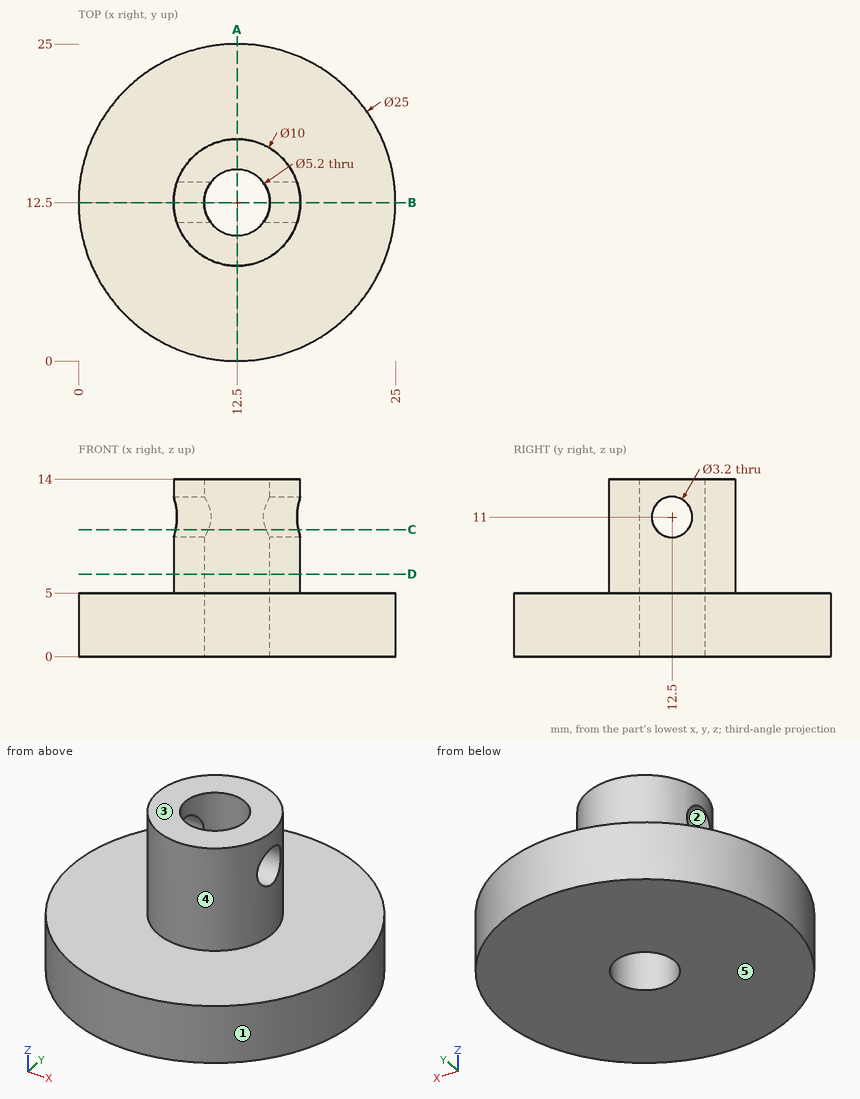
Geometry check sheet. Reference: drawing and pictorial views, mm from the part's lowest x, y, z. A direction names the side the tool comes from. Round coordinates to 2 decimals unless told otherwise and drop trailing zeros. Order: outer loops, then holes, each group sorted by start corner. A loop starts at its lowest first (then second) coordinate and runs counter-clockwise, first axis right, second up. Notation, with made-up numbers: (-21.75, -1) - (-0.75, -1) arc R5 ccw to (-0.75, 8) - close; hole circle Ø5 at (-24.5, 58). An arc over 180 degrees is marked (long way). One line per question, with ' | ' between items. Start each with the question number.
(1) Sectioned sample at D-D on z = 6.5. Record the cut outline in (x, y).
(2) Access from +Z, -Z, +X, -X, +Y, -Y to the whole of each face (thin tool, end or side, straight path). Record for the marked faces 4 and 5.
(3) Thickness scan on L1, parallel to Z at x = 15.3, y = 12.5; L2, parallel to X at y = 14.5, z = 9.75; L3, parallel to Z at x = 7.25, y = 21.25. Record the ranges inside material, lowest first. Write a range as [from, to].
(4) Sectioned sample at B-B on y = 12.5. Record the cut outline in (x, z).
(5) Sectioned sample at A-A on x = 12.5. Record the cut outline in (y, z), and give its area (3 significant figures).
(6) Depth check by flat-ended pin: pin 1 Ø8 at (y, z) = (22.5, 5) entering from +X; pin 2 Ø6 at (y, z) = (21, 6.5) entering from -X; pin 3 Ø6 at (x, z) = (18, 11) entering from -Y. Enter the tip coordinate at first touch or a pass-through.
(7) Sectioned sample at C-C on z = 10. Record the cut outline in (x, y).
(8) Release check for a two-part mould opening along Z. For the marked faces 1, 2 and 3 record: released by +Z, released by -Z, zero draft, split by the parting line, or undercut.
Conclusion:
1) outline: circle Ø10 at (12.5, 12.5); hole circle Ø5.2 at (12.5, 12.5)
2) face 4: +Z | face 5: -Z, +X, -X, +Y, -Y
3) L1: z = [0, 9.4], [12.6, 14] | L2: x = [7.92, 10.84], [14.16, 17.08] | L3: z = [0, 5]
4) outline: (0, 0) - (9.9, 0) - (9.9, 9.4) - (7.5, 9.4) - (7.5, 5) - (0, 5) - close; (7.5, 12.6) - (9.9, 12.6) - (9.9, 14) - (7.5, 14) - close; (15.1, 0) - (25, 0) - (25, 5) - (17.5, 5) - (17.5, 9.4) - (15.1, 9.4) - close; (15.1, 12.6) - (17.5, 12.6) - (17.5, 14) - (15.1, 14) - close
5) outline: (0, 0) - (9.9, 0) - (9.9, 14) - (7.5, 14) - (7.5, 5) - (0, 5) - close; (15.1, 0) - (25, 0) - (25, 5) - (17.5, 5) - (17.5, 14) - (15.1, 14) - close | area: 142 mm2
6) pin 1: stops at x = 23.47 | pin 2: stops at x = 1.48 | pin 3: stops at y = 8.17
7) outline: (7.66, 11.25) arc R5 ccw to (17.34, 11.25) - (14.78, 11.25) arc R2.6 cw to (10.22, 11.25) - close; (7.66, 13.75) - (10.22, 13.75) arc R2.6 cw to (14.78, 13.75) - (17.34, 13.75) arc R5 ccw to start
8) face 1: zero draft | face 2: undercut | face 3: released by +Z
